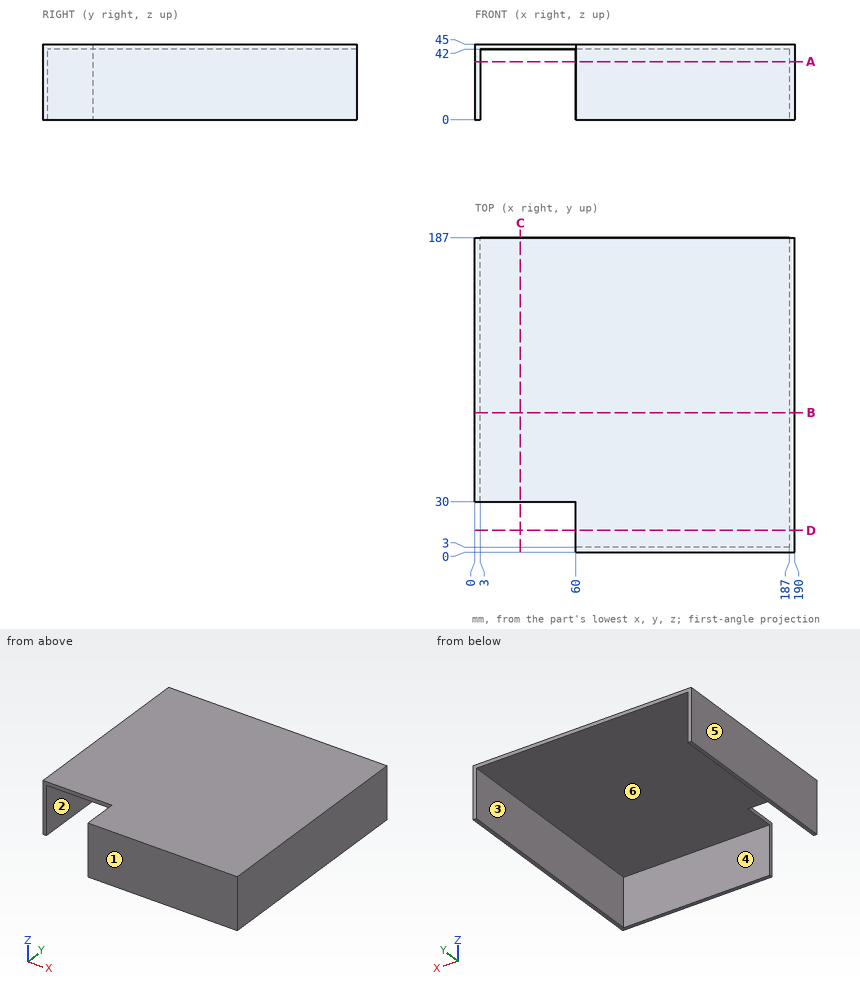
Can you work these out from the drawing? Everything is in mm from the part's minimum corner. A direction names the side the tool comes from. Coordinates: 2 decimals unless noted, no trailing zeros. Loops run counter-clockwise (first coordinate to the right, second up) from the corner with the lowest first, then second, coordinate; pieces in that order, holes last.
1) For pin 1 (6 mm diameter, centred on x = 107, y = 50, fed in from -Z); pin 2 (1.5 mm diameter, centred on x = 59, z = 37.5, fed in from -Y); pin 3 (9 mm diameter, centred on y = 19, z = 14.5, fed in from -X); pin 4 (21 mm diameter, centred on x = 135, z = 12, fed in from +Y), each with a flat end and sliding along its axis, tell me the tip position at first contact or that it passes through.
2) I need wall thicknesses on probe 1 along X at (y, z) = (175, 22.5); probe 2 along Z at (x, y) = (22, 152.5); probe 3 along Y at (x, z) = (101.5, 16). Which ranges of each line are inside material? Lowest first, please.
3) Imagine slicing it at C-C on x = 27. List the corners of the cut face in (y, z) for me, plus the area to 3 significant figures.
4) Imagine slicing it at A-A on z = 34.5. List the corners of the cut face in (x, y) for me.
5) Thinking about a two-plate mould opening in X: for the marked faces 4, 5 and 6, which applies, pulls with the +X half, pulls with the -X half, needs draft (parallel to the pull), parting line crosses it, or undercut?
6) Imagine slicing it at B-B on y = 83. List the corners of the cut face in (x, z) for me, plus the area to 3 significant figures.
7) Imagine slicing it at D-D on y = 13. List the corners of the cut face in (x, z) for me, plus the area to 3 significant figures.
8) Which directions (+Z, -Z, +X, -X, +Y, -Y) give clear straight access to the entire face, cutting with the end or side of a thin tool? Please do the marked faces 1, 2 and 3.
Completed:
1. pin 1: stops at z = 42
1. pin 2: passes through
1. pin 3: stops at x = 187
1. pin 4: stops at y = 3
2. probe 1: x = 0 to 3, 187 to 190
2. probe 2: z = 42 to 45
2. probe 3: y = 0 to 3
3. outline: (30, 42) - (187, 42) - (187, 45) - (30, 45) - close
3. area: 471 mm2
4. outline: (0, 30) - (3, 30) - (3, 187) - (0, 187) - close; (60, 0) - (190, 0) - (190, 187) - (187, 187) - (187, 3) - (60, 3) - close
5. face 4: needs draft
5. face 5: pulls with the -X half
5. face 6: undercut
6. outline: (0, 0) - (3, 0) - (3, 42) - (187, 42) - (187, 0) - (190, 0) - (190, 45) - (0, 45) - close
6. area: 822 mm2
7. outline: (60, 42) - (187, 42) - (187, 0) - (190, 0) - (190, 45) - (60, 45) - close
7. area: 516 mm2
8. face 1: +Z, -Z, +X, -X, -Y
8. face 2: -Z, +Y, -Y
8. face 3: -Z, +Y
